Read the model definition and answer for the solid it produces. Units are mm, in the model's axes. Give positions to 0.01 mm unless a question says otherwise; leave off trailing zeros. Order: outer loops, then holes, each group sorted by start corner. A loop starts at its lowest first (then second) coordinate and runs counter-clockwise, first axis right, second up. Notation, with made-up numbers: (-36, 64) -> (-14, 64) arc R27 cw to (-14, 92) -> close; hole circle Ø1 at (-38.75, 63.5). An arc over 180 degrees is marked (long way). One line per item, written item: value. Start each with the question number.
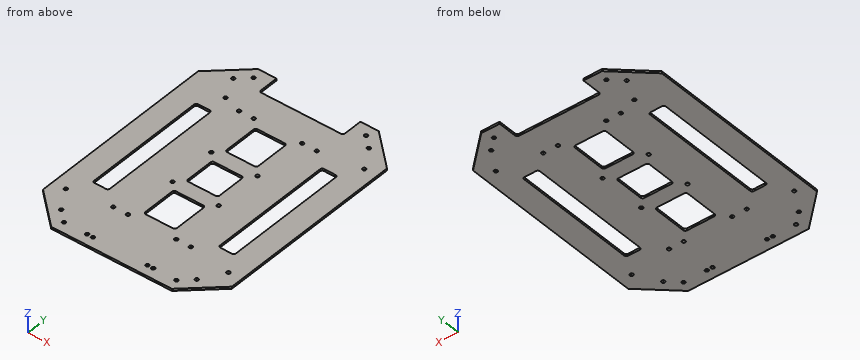
from build123d import *

# Parameters (mm, degrees)
F0_W     = 180
F0_H     = 180
F1_DEPTH = 2
F2_D     = 3.3
F4_D     = 3.3
F6_D     = 3.3
F7_W     = 30
F7_H     = 30
F7_H_2   = 35
F7_W_2   = 15
F7_H_3   = 120
F7_W_3   = 80
F7_H_4   = 20
F8_DEPTH = 2.001
F9_R     = 2


with BuildPart() as f1:
    # F0 (on Top) → F1 (new body)
    with BuildSketch(Plane.XY):
        Rectangle(F0_W, F0_H)
        Polygon((-90, 90), (90, 90), (57.5, 120), (-57.5, 120), align=None)
        Polygon((57.5, -120), (90, -90), (-90, -90), (-57.5, -120), align=None)
    extrude(amount=F1_DEPTH)

    # F2 (through all)
    with Locations(Plane(origin=(0, 0, 0), x_dir=(1, 0, 0), z_dir=(0, 0, -1))):
        with Locations((-23, -73), (23, -73), (23, 73), (-23, 73), (-54.58, -78.75), (37, -73), (77.5, -78.75), (-77.5, 78.75), (-37, 73), (77.5, 78.75), (37, 73), (-37, -73)):
            Hole(F2_D / 2)

    # F4 (through all)
    with Locations(Plane(origin=(0, 0, 0), x_dir=(1, 0, 0), z_dir=(0, 0, -1))):
        with Locations((-64.6122133253, 99.825798459), (-53.5901616559, 110), (53.5901616559, 110), (64.6122133253, 99.825798459), (64.6122133253, -99.825798459), (53.5901616559, -110), (-53.5901616559, -110), (-64.6122133253, -99.825798459)):
            Hole(F4_D / 2)

    # F6 (through all)
    with Locations(Plane(origin=(0, 0, 0), x_dir=(1, 0, 0), z_dir=(0, 0, -1))):
        with Locations((-22, -22.5), (22, -22.5), (22, 22.5), (-22, 22.5), (25.9754041397, 110), (31.4754041397, 110), (-25.9754041397, 110), (-31.4754041397, 110)):
            Hole(F6_D / 2)

    # F7 (on Top) → F8 (cut, through all)
    with BuildSketch(Plane.XY):
        Rectangle(F7_W, F7_H)
        with Locations((0, 47.5)):
            Rectangle(F7_W, F7_H_2)
        with Locations((0, -47)):
            Rectangle(F7_W, F7_H_2)
        with Locations((-60, 0)):
            Rectangle(F7_W_2, F7_H_3)
        with Locations((60, 0)):
            Rectangle(F7_W_2, F7_H_3)
        with Locations((0, 110)):
            Rectangle(F7_W_3, F7_H_4)
    extrude(amount=F8_DEPTH, mode=Mode.SUBTRACT)

    # F9
    f9_edges = [f1.edges().sort_by_distance(p)[0] for p in [
        (-52.5, -60, 1),
        (-67.5, -60, 1),
        (-52.5, 60, 1),
        (15, 65, 1),
        (15, 15, 1),
        (15, -29.5, 1),
        (67.5, 60, 1),
        (15, 30, 1),
        (15, -15, 1),
        (67.5, -60, 1),
        (40, 100, 1),
        (15, -64.5, 1),
        (-67.5, 60, 1),
        (-15, 65, 1),
        (-15, 15, 1),
        (-15, -29.5, 1),
        (52.5, -60, 1),
        (-15, -64.5, 1),
        (-40, 100, 1),
        (-15, -15, 1),
        (-15, 30, 1),
        (52.5, 60, 1),
    ]]
    fillet(f9_edges, radius=F9_R)


solid = f1.part
Item 1: Flat-ended cylindrical pins translate along their axes: pin 1 (4.5 mm diameter, centred on x = 77.5, y = -78.75, fed in from +Z); pin 2 (3 mm diameter, centred on x = -25.98, y = -110, fed in from -Z). Find the tip coordinate at first contact, or state that the pin passes through.
Item 2: Find section A-A on y = -2. Write down the section's boundary in (x, z).
Item 3: Find section B-B on x = -9.5. Write down the section's boundary in (y, z), then the cut area to 3 significant figures.
Item 4: Find the intervals of material crossed by line 1 (X direction, y = 47, z = 0.4); line 2 (X direction, y = 22.5, z = 1.3); line 3 (X direction, y = -17, z = 1.15), in increasing order. Write a range as from..to.
Item 5: Find section C-C on z = 1.05. Count the separate pieces of the cut face and the enclosed holes in it, then the cut area to 3 significant figures.
Checks:
1. pin 1: z = 2
1. pin 2: through
2. outline: (-90, 0) -> (-67.5, 0) -> (-67.5, 2) -> (-90, 2) -> close; (-52.5, 0) -> (-15, 0) -> (-15, 2) -> (-52.5, 2) -> close; (15, 0) -> (52.5, 0) -> (52.5, 2) -> (15, 2) -> close; (67.5, 0) -> (90, 0) -> (90, 2) -> (67.5, 2) -> close
3. outline: (-120, 0) -> (-64.5, 0) -> (-64.5, 2) -> (-120, 2) -> close; (-29.5, 0) -> (-15, 0) -> (-15, 2) -> (-29.5, 2) -> close; (15, 0) -> (30, 0) -> (30, 2) -> (15, 2) -> close; (65, 0) -> (100, 0) -> (100, 2) -> (65, 2) -> close
3. area: 240 mm2
4. line 1: -90..-67.5, -52.5..-15, 15..52.5, 67.5..90
4. line 2: -90..-67.5, -52.5..-23.65, -20.35..20.35, 23.65..52.5, 67.5..90
4. line 3: -90..-67.5, -52.5..52.5, 67.5..90
5. separate pieces: 1
5. enclosed holes: 33
5. area: 32,800 mm2
